For this review, take the finished solid that the model builds, in its own axes (mm). A direction names the side the tool comes from. Give positions to 0.01 mm unless a question says otherwise; leave off trailing zeros. Loops run counter-clockwise (first coordinate to the right, second up) from the corner with the lowest first, then second, coordinate; pieces in that order, holes last. Notation, with made-up numbers: (-3, 26.25) - (26, 26.25) arc R22 cw to (26, 51.25) - close; hole circle Ø3 at (-29, -2.75). An arc over 180 degrees is marked (long way). Put each result on its own line as item: value. Start each with the question number.
from build123d import *

# Parameters (mm, degrees)
SKETCH1_R               = 1.5
BOSS_EXTRUDE1_DEPTH     = 5
CUT_EXTRUDE1_DEPTH      = 37
CUT_EXTRUDE1_DEPTH_BACK = 24
SKETCH2_R               = 5


with BuildPart() as part:
    # Sketch1 → Boss-Extrude1 (new body)
    with BuildSketch(Plane.XY):
        with BuildLine():
            Line((-20, -76.707766284), (-20, -58.504148974))
            Line((-20, -58.504148974), (-150, -58.504148974))
            Line((-150, -58.504148974), (-150, -33.504148974))
            Line((-150, -33.504148974), (-20, -34.707766284))
            Line((-20, -34.707766284), (20, -34.707766284))
            Line((20, -34.707766284), (20, -76.707766284))
            ThreePointArc((20, -76.707766284), (0, -96.707766284), (-20, -76.707766284))
        make_face()
        with Locations((0, -44.707766284)):
            Circle(SKETCH1_R, mode=Mode.SUBTRACT)
        with Locations((-130, -43.689749466)):
            Circle(SKETCH1_R, mode=Mode.SUBTRACT)
    extrude(amount=BOSS_EXTRUDE1_DEPTH)

    # Sketch2 → Cut-Extrude1 (cut, two sides: drawn at the far end of the back side and taken through both)
    with BuildSketch(Plane.XY.offset(5).offset(-CUT_EXTRUDE1_DEPTH_BACK)):
        with Locations((0, -74.90788056)):
            Circle(SKETCH2_R)
    extrude(amount=CUT_EXTRUDE1_DEPTH + CUT_EXTRUDE1_DEPTH_BACK, mode=Mode.SUBTRACT)


solid = part.part
1) Take a section at D-D on y = -62.5. State the section outline as (x, z) points.
2) Take a section at C-C on z = 3.7. State the section outline as (x, y) points, and give its area (3 significant figures).
3) Take a section at A-A on x = 0. State the section outline as (y, z) points, and give its area (3 significant figures).
4) Mouldability with a two-part tool opening along X and no side actions: class faces 1 (the flat face through (-45, -51, 0)), 2 (the flat face through (20, -55, 2)), 3 (the cylindrical face through (-1.08, -79.79, 2.46)), 4 (the flat face through (-150, -46, 2)) as released by +X, released by -X, zero draft, split by the parting line, or undercut.
5) Insertion check: P1, Ø2.5, axis at x = -130, y = -43.69, coming from the +Z side; P2, Ø2, axis at x = -64, y = -49, coming from the -Z side; P3, Ø1.5, axis at y = -69.5, z = 3, coming from the -X side; P4, Ø1.5, axis at x = 3, z = 2, coming from the +Y side. Each pin has a flat end and moves straight along its axis. Give the tip position at first contact, or say it passes through.
6) Wall thickness on probe 1 along Y at (x, z) = (0, 1.2); probe 2 along X at (y, z) = (-60, 2.1); probe 3 along Y at (x, z) = (-130, 1.8): over which ranges is each line inside the solid? List them lowest first.
7) Machinability: for faces 5 (the flat face through (-20, -68, 2)), 6 (the flat face through (0, -34.708, 2)), 7 (the cylindrical face through (-0.33, -46.17, 2.46)), which of the approach directions +Z, -Z, +X, -X, +Y, -Y give a long, thin tool a straight path to every point of the face, cutting with its end or side? Answer none if there is none.
8) Take a section at B-B on x = -130. State the section outline as (y, z) points, and give its area (3 significant figures).
Answers follow:
1. outline: (-20, 0) - (20, 0) - (20, 5) - (-20, 5) - close
2. outline: (-150, -58.5) - (-20, -58.5) - (-20, -76.71) arc R20 ccw to (20, -76.71) - (20, -34.71) - (-20, -34.71) - (-150, -33.5) - close; hole circle Ø3 at (-130, -43.69); hole circle Ø10 at (0, -74.91); hole circle Ø3 at (0, -44.71)
2. area: 5,390 mm2
3. outline: (-96.71, 0) - (-79.91, 0) - (-79.91, 5) - (-96.71, 5) - close; (-69.91, 0) - (-46.21, 0) - (-46.21, 5) - (-69.91, 5) - close; (-43.21, 0) - (-34.71, 0) - (-34.71, 5) - (-43.21, 5) - close
3. area: 245 mm2
4. face 1: zero draft
4. face 2: released by +X
4. face 3: undercut
4. face 4: released by -X
5. P1: through
5. P2: z = 0
5. P3: x = -20
5. P4: y = -34.71
6. probe 1: -96.71 to -79.91, -69.91 to -46.21, -43.21 to -34.71
6. probe 2: -20 to 20
6. probe 3: -58.5 to -45.19, -42.19 to -33.69
7. face 5: +Z, -Z, -X, -Y
7. face 6: +Z, -Z, +X, +Y
7. face 7: +Z, -Z
8. outline: (-58.5, 0) - (-45.19, 0) - (-45.19, 5) - (-58.5, 5) - close; (-42.19, 0) - (-33.69, 0) - (-33.69, 5) - (-42.19, 5) - close
8. area: 109 mm2
